from build123d import *

# Parameters (mm, degrees)
F1_DEPTH = 180
F2_T     = -3


with BuildPart() as f1:
    # F0 (on Right) → F1 (new body)
    with BuildSketch(Plane.YZ):
        Polygon((-251, 46), (-251, -46), (251, -46), (391, 46), (251, 46), align=None)
    extrude(amount=F1_DEPTH)

    # F2
    f2_openings = [f1.faces().sort_by_distance(p)[0] for p in [
        (90, 70, 46),
    ]]
    offset(amount=F2_T, openings=f2_openings)


solid = f1.part
Input: part model. Units: mm. Frame: model coordinates. A direction names the side the tool comes from. Give positions to 0.01 mm unless a question says otherwise; leave off trailing zeros. Loops run counter-clockwise (first coordinate to the right, second up) from the corner with the lowest first, then second, coordinate; pieces in that order, holes last. Notation, with made-up numbers: (38.5, 52.5) -> (94.5, 52.5) arc R16 ccw to (94.5, 57.5) -> close; hole circle Ø10 at (78.25, -26.5). An arc over 180 degrees is marked (long way). Answer as a JSON object with one key per item and string values. Group by question number.
Item 1: Pin query (flat end, axial travel): P1, Ø12, axis at x = 34, z = 11, coming from the +Y side; P2, Ø6, axis at x = 134.5, y = 218, coming from the +Z side; P3, Ø3, axis at y = -172, z = 26.5, coming from the -X side; P4, Ø6, axis at x = 109.5, y = 295, coming from the -Z side. Return the tip coordinate at first contact, or that it passes through.
Item 2: Cut plane A-A, the plane z = 38.5. Return the cut outline in (x, y), and give its area (3 significant figures).
Item 3: Reachability of faces 4 (the flat face through (89, -251, 1)), 5 (the flat face through (3, 64, 2)) from +Z, -Z, +X, -X, +Y, -Y: full face, straight path, thin tool, end or side. Return the list, or none.
Item 4: Cut plane D-D, the plane z = -12. Return the cut outline in (x, y), and give its area (3 significant figures).
Item 5: Pull-direction query (X, two-part tool) for faces 1 (the flat face through (89, -248, 2)), 2 (the flat face through (89, -4, -46)), 3 (the flat face through (180, 66, 1)); classes: released by +X, released by -X, zero draft, split by the parting line, or undercut.
Item 6: Cut plane C-C, the plane y = 109.5. Return the cut outline in (x, z), and give its area (3 significant figures).
Item 7: Cut plane B-B, the plane x = 139. Return the cut outline in (y, z).
Item 8: Line query: probe 1 along X at (y, z) = (-145, 15); probe 2 along Y at (x, z) = (103.5, 36.5); probe 3 along Z at (x, y) = (21, 150). Output: solid intervals per line, ascending.
Checks:
{
 "1": {"P1": "stops at y = 346.87", "P2": "stops at z = -43", "P3": "stops at x = 0", "P4": "stops at z = -19.06"},
 "2": {"outline": "(0, -251) -> (180, -251) -> (180, 379.59) -> (0, 379.59) -> close; hole (3, -248) -> (177, -248) -> (177, 374.12) -> (3, 374.12) -> close", "area": "5,260 mm²"},
 "3": {"face 4": "+Z, -Z, +X, -X, -Y", "face 5": "+Z"},
 "4": {"outline": "(0, -251) -> (180, -251) -> (180, 302.74) -> (0, 302.74) -> close; hole (3, -248) -> (177, -248) -> (177, 297.28) -> (3, 297.28) -> close", "area": "4,790 mm²"},
 "5": {"face 1": "undercut", "face 2": "zero draft", "face 3": "released by +X"},
 "6": {"outline": "(0, -46) -> (180, -46) -> (180, 46) -> (177, 46) -> (177, -43) -> (3, -43) -> (3, 46) -> (0, 46) -> close", "area": "1,070 mm²"},
 "7": {"outline": "(-251, -46) -> (251, -46) -> (391, 46) -> (385.54, 46) -> (250.1, -43) -> (-248, -43) -> (-248, 46) -> (-251, 46) -> close"},
 "8": {"probe 1": "x = 0 to 3, 177 to 180", "probe 2": "y = -251 to -248, 371.08 to 376.54", "probe 3": "z = -46 to -43"}
}
